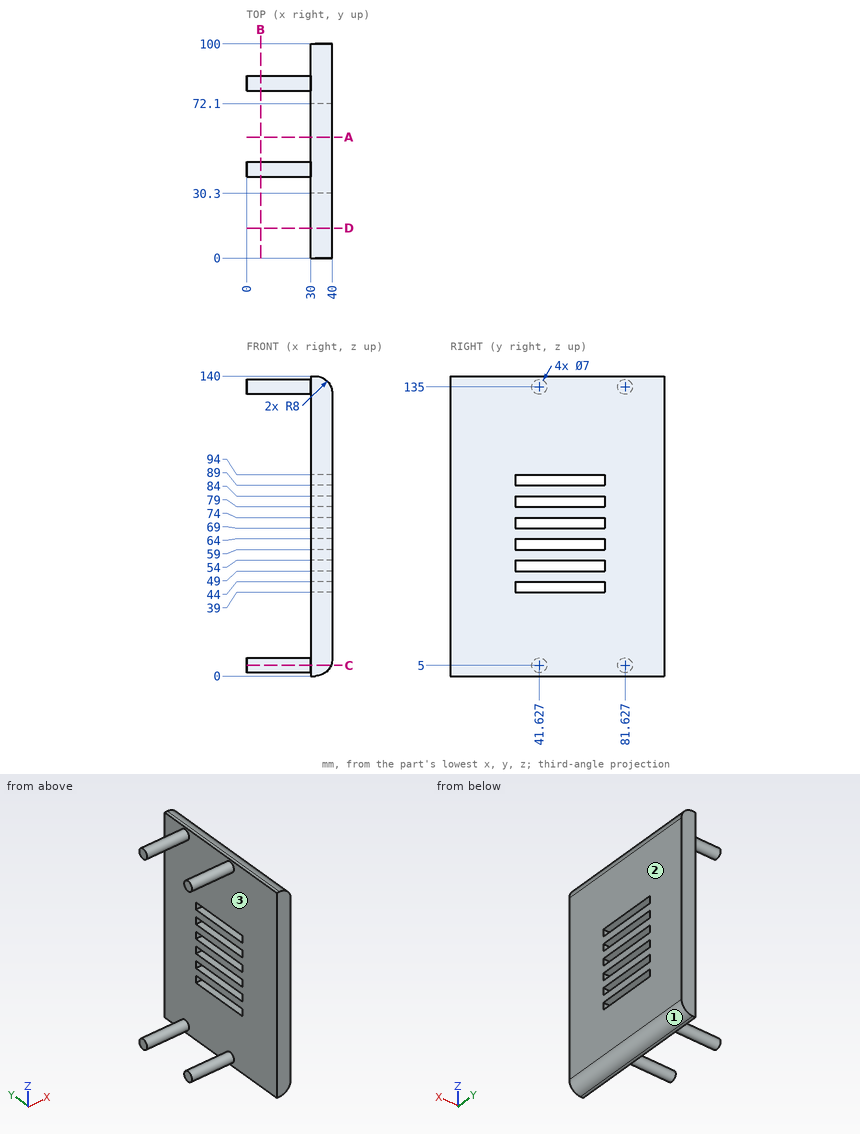
Could you check a few things on this drawing? It's one solid part, dimensions in mm from its lowest x, y, z. Give positions to 0.01 mm unless a question says otherwise; leave off trailing zeros. Order: outer loops, then holes, each group sorted by start corner. A loop starts at its lowest first (then second) coordinate and runs counter-clockwise, first axis right, second up. Notation, with made-up numbers: (-24, 29) - (31, 29) arc R20 ccw to (31, 66) - close; hole circle Ø10 at (84.25, 42). An arc over 180 degrees is marked (long way). Return JSON: item names as keys, results as strings. Group by question number.
Q1. Suppose I cut it at D-D, the plane y = 14. Please give me the cut outline in (x, z).
Q2. Will these pins go through, and if not, where does the flat tip stop? pin 1 Ø12 at (y, z) = (24, 80.5) entering from -X; pin 2 Ø3 at (x, y) = (37.5, 55.5) entering from -Z; pin 3 Ø3 at (x, y) = (35.5, 51.5) entering from +Z.
Q3. Suppose I cut it at A-A, the plane y = 56.5. State how many separate pieces and enclosed holes the cut face has, and give its area (3 significant figures).
Q4. Suppose I cut it at C-C, the plane z = 5. Please give me the cut outline in (x, y), and give its area (3 significant figures).
Q5. Please list where these lines run through material, in increasing order: line 1 along X through (y, z) = (16, 88); line 2 along Z through (x, y) = (11.5, 81); line 3 along Z through (x, y) = (17.5, 40.5). Write a range as [from, to].
Q6. Thinking about a two-plate mould opening in Z: for the marked faces 1, 2 and 3, which applies, pulls with the +Z half, pulls with the -Z half, needs draft (parallel to the pull), parting line crosses it, or undercut?
Q7. Suppose I cut it at B-B, the plane x = 6.5. Please give me the cut outline in (y, z), and give its area (3 significant figures).
Resolved:
{
 "1": {"outline": "(30, 0) - (32, 0) arc R8 ccw to (40, 8) - (40, 132) arc R8 ccw to (32, 140) - (30, 140) - close"},
 "2": {"pin 1": "stops at x = 30", "pin 2": "stops at z = 1.07", "pin 3": "stops at z = 139.75"},
 "3": {"separate pieces": "7", "enclosed holes": "0", "area": "1,070 mm2"},
 "4": {"outline": "(0, 38.13) - (30, 38.13) - (30, 0) - (39.42, 0) - (39.42, 100) - (30, 100) - (30, 85.13) - (0, 85.13) - (0, 78.13) - (30, 78.13) - (30, 45.13) - (0, 45.13) - close", "area": "1,360 mm2"},
 "5": {"line 1": "x = [30, 40]", "line 2": "z = [1.56, 8.44], [131.56, 138.44]", "line 3": "z = [1.69, 8.31], [131.69, 138.31]"},
 "6": {"face 1": "pulls with the -Z half", "face 2": "needs draft", "face 3": "undercut"},
 "7": {"outline": "circle Ø7 at (41.63, 5); circle Ø7 at (41.63, 135); circle Ø7 at (81.63, 5); circle Ø7 at (81.63, 135)", "area": "154 mm2"}
}
